Geometry: final body of the model. Coordinates: model frame, mm. Face numbers are marked on the shaded views. Give positions to 0.01 mm unless a question says otherwise; leave off trailing zeros. Loops run counter-clockwise (first coordinate to the right, second up) from the corner with the lowest first, then second, coordinate; pieces in that order, holes last. Notation, with made-up numbers: (13, 8) -> (42, 8) arc R22 ccw to (42, 19) -> close; hole circle Ø3 at (-14, 53). An arc over 180 degrees is marked (long way). One line per question, with ' | ' between items. Start each with the question number.
Item 1: Section C-C on x = -17.5. Return loops of the section in (y, z).
Item 2: Section B-B on z = 43.5. Return loops of the section in (x, y).
Item 3: Mould query, pull axis Y, two halves, no side actions, for the marked faces 1, 2 and 3. Classes: released by +Y, released by -Y, zero draft, split by the parting line, or undercut.
Item 4: Section A-A on y = -117.5. Return loops of the section in (x, z).
Item 5: Material intervals for line 1 along X through (y, z) = (-138, 7); line 2 along Z through (x, y) = (61, -156); line 3 along Z through (x, y) = (2.5, -124.5), sorted ascending. Write a range as [from, to].
Item 6: Pin query (flat end, axial travel): P1, Ø6, axis at y = 0, z = 33, coming from the -X side; P2, Ø4.5, axis at y = -1, z = 29.5, coming from the +X side; P3, Ø4, axis at x = 45.5, y = -101.5, coming from the +Z side; P4, Ø3.5, axis at x = 0, z = 23.49, coming from the +Y side. Return the tip coordinate at first contact, or that it passes through.
Item 7: Section D-D on z = 9. Return loops of the section in (x, y), then the cut area to 3 significant figures.
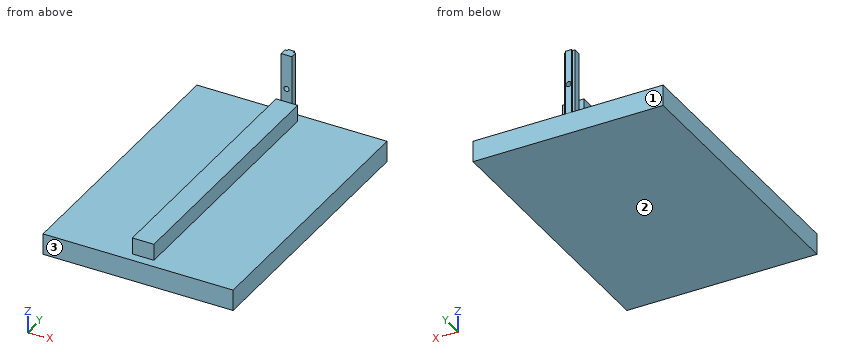
from build123d import *

# Parameters (mm, degrees)
F0_W     = 2.342829
F0_H     = 1.397
F0_W_2   = 2.34442
F1_DEPTH = 50.8
F3_D     = 4.064
F4_W     = 16.880292
F4_H     = 12.94488
F5_DEPTH = 203.2
F6_W     = 148.601494
F6_H     = 217.50565
F7_DEPTH = 16.51


with BuildPart() as f1:
    # F0 (on Top) → F1 (new body)
    with BuildSketch(Plane.XY):
        Polygon((-4.1275, -2.794), (4.1275, -2.794), (4.1275, 2.794), (2.9845, 2.794), (2.35712, 2.794), (0.0127, 2.794), (-0.0127, 2.794), (-2.355529, 2.794), (-4.1275, 2.794), align=None)
        with Locations((-1.184114, 3.4925)):
            Rectangle(F0_W, F0_H)
        with Locations((1.18491, 3.4925)):
            Rectangle(F0_W_2, F0_H)
        Polygon((-0.0127, 4.191), (-0.0127, 2.794), (0.0127, 2.794), (0.0127, 4.191), (0, 4.191), align=None)
    extrude(amount=F1_DEPTH)

    # F3 (through all)
    with Locations(Plane.XZ.offset(2.794)):
        with Locations((0, 23.493898)):
            Hole(F3_D / 2)

    # F4 (on face) → F5 (join)
    with BuildSketch(Plane.XZ.offset(2.794)):
        with Locations((0.316053, 6.454206)):
            Rectangle(F4_W, F4_H)
    extrude(amount=F5_DEPTH)

    # F6 (on face) → F7 (join)
    with BuildSketch(Plane(origin=(0, 0, -0.018234), x_dir=(1, 0, 0), z_dir=(0, 0, -1))):
        with Locations((0.316053, 104.394)):
            Rectangle(F6_W, F6_H)
    extrude(amount=F7_DEPTH)


solid = f1.part
Result sheet:
1) outline: (-213.15, -16.53) -> (4.36, -16.53) -> (4.36, -0.02) -> (-213.15, -0.02) -> close
2) outline: (-4.13, -2.79) -> (4.13, -2.79) -> (4.13, 2.79) -> (2.36, 2.79) -> (2.36, 4.19) -> (-2.36, 4.19) -> (-2.36, 2.79) -> (-4.13, 2.79) -> close
3) face 1: released by +Y | face 2: zero draft | face 3: released by -Y
4) outline: (-73.98, -16.53) -> (74.62, -16.53) -> (74.62, -0.02) -> (8.76, -0.02) -> (8.76, 12.93) -> (-8.12, 12.93) -> (-8.12, -0.02) -> (-73.98, -0.02) -> close
5) line 1: x = [-8.12, 8.76] | line 2: z = [-16.53, -0.02] | line 3: z = [-16.53, 12.93]
6) P1: stops at x = -4.13 | P2: stops at x = 4.13 | P3: stops at z = -0.02 | P4: passes through
7) outline: (-8.12, -205.99) -> (8.76, -205.99) -> (8.76, -2.79) -> (4.13, -2.79) -> (4.13, 2.79) -> (2.36, 2.79) -> (2.36, 4.19) -> (-2.36, 4.19) -> (-2.36, 2.79) -> (-4.13, 2.79) -> (-4.13, -2.79) -> (-8.12, -2.79) -> close | area: 3,480 mm²
